Work out the finished part from the listing and answer in its coordinate system (mm). Round coordinates to 2 decimals unless told otherwise and drop trailing zeros. Write each loop counter-clockwise with the first axis right and the second up, starting at its lowest first coordinate (ties: lowest second). Pieces come first, ordered by that corner, then holes.
1. Find section D-D (x = -0.5). Write down the section's boundary in (y, z), and give its area (3 significant figures).
2. Find section B-B (x = 33.5). Write down the section's boundary in (y, z), and give its area (3 significant figures).
3. Find section A-A (z = 5.75). Count the separate pieces of the cut face and the enclosed holes in it, and give its area (3 significant figures).
4. Find section C-C (y = -5.25). Write down the section's boundary in (x, z).
5. Straight lines are drawn through the part: probe 1 along X at (y, z) = (-2, 2.25); probe 2 along Y at (x, z) = (8, 5.75); probe 3 along X at (y, z) = (-6.25, 5.25). For each, find the intervals that lie inside material, in ascending order.
6. Flat-ended cylindrical pins translate along their axes: pin 1 Ø3 at (y, z) = (-1.5, 4) entering from +X; pin 2 Ø1.5 at (y, z) = (-2, 5.5) entering from +X. Find the tip coordinate at first contact, or state that the pin passes through.
7. Determine the mould class of faces 1 (the face through (16, -1, 0)), 2 (the face through (26.16, -4.94, 3.91)), 3 (the face through (35.718, -4.056, 3.913)), 4 (the face through (-3.968, -3.881, 3.913)) for opening direction X: pulls with the +X half, pulls with the -X half, needs draft (parallel to the pull), parting line crosses it, or undercut.
```python
from build123d import *

# Parameters (mm, degrees)
F0_R     = 2.54
F1_DEPTH = 7.9375


with BuildPart() as f1:
    # F0 (on Top) → F1 (new body)
    with BuildSketch(Plane.XY):
        with BuildLine():
            Line((31.75, 0), (0, 0))
            Line((0, 0), (0, -1.42875))
            ThreePointArc((0, -1.42875), (1.796051, -2.172699), (2.54, -3.96875))
            ThreePointArc((2.54, -3.96875), (1.796051, -5.764801), (0, -6.50875))
            Line((0, -6.50875), (0, -7.9375))
            Line((0, -7.9375), (31.75, -7.9375))
            Line((31.75, -7.9375), (31.75, -6.50875))
            ThreePointArc((31.75, -6.50875), (29.21, -3.96875), (31.75, -1.42875))
            Line((31.75, -1.42875), (31.75, 0))
        make_face()
        with Locations((7.9375, -3.96875)):
            Circle(F0_R, mode=Mode.SUBTRACT)
        with Locations((15.875, -3.96875)):
            Circle(F0_R, mode=Mode.SUBTRACT)
        with Locations((23.8125, -3.96875)):
            Circle(F0_R, mode=Mode.SUBTRACT)
        with BuildLine():
            Line((0, -1.42875), (0, 0))
            ThreePointArc((0, 0), (-3.96875, -3.96875), (0, -7.9375))
            Line((0, -7.9375), (0, -6.50875))
            ThreePointArc((0, -6.50875), (-2.54, -3.96875), (0, -1.42875))
        make_face()
        with BuildLine():
            ThreePointArc((31.75, -7.9375), (35.71875, -3.96875), (31.75, 0))
            Line((31.75, 0), (31.75, -1.42875))
            ThreePointArc((31.75, -1.42875), (33.546051, -2.172699), (34.29, -3.96875))
            ThreePointArc((34.29, -3.96875), (33.546051, -5.764801), (31.75, -6.50875))
            Line((31.75, -6.50875), (31.75, -7.9375))
        make_face()
    extrude(amount=F1_DEPTH)


solid = f1.part
```
Worked answers:
1. outline: (-7.91, 0) - (-6.46, 0) - (-6.46, 7.94) - (-7.91, 7.94) - close; (-1.48, 0) - (-0.03, 0) - (-0.03, 7.94) - (-1.48, 7.94) - close
1. area: 23.0 mm2
2. outline: (-7.53, 0) - (-5.81, 0) - (-5.81, 7.94) - (-7.53, 7.94) - close; (-2.13, 0) - (-0.41, 0) - (-0.41, 7.94) - (-2.13, 7.94) - close
2. area: 27.3 mm2
3. separate pieces: 1
3. enclosed holes: 5
3. area: 200 mm2
4. outline: (-3.76, 0) - (-2.19, 0) - (-2.19, 7.94) - (-3.76, 7.94) - close; (2.19, 0) - (5.74, 0) - (5.74, 7.94) - (2.19, 7.94) - close; (10.13, 0) - (13.68, 0) - (13.68, 7.94) - (10.13, 7.94) - close; (18.07, 0) - (21.62, 0) - (21.62, 7.94) - (18.07, 7.94) - close; (26.01, 0) - (29.56, 0) - (29.56, 7.94) - (26.01, 7.94) - close; (33.94, 0) - (35.51, 0) - (35.51, 7.94) - (33.94, 7.94) - close
5. probe 1: x = -3.45 to -1.6, 1.6 to 6.33, 9.54 to 14.27, 17.48 to 22.21, 25.42 to 30.15, 33.35 to 35.2
5. probe 2: y = -7.94 to -6.51, -1.43 to 0
5. probe 3: x = -3.25 to -1.12, 1.12 to 6.82, 9.05 to 14.76, 16.99 to 22.7, 24.93 to 30.63, 32.87 to 35
6. pin 1: stops at x = 35.6
6. pin 2: stops at x = 35.53
7. face 1: needs draft
7. face 2: undercut
7. face 3: pulls with the +X half
7. face 4: pulls with the -X half
